Verification items for the finished model (mm, model axes). A direction names the side the tool comes from. Coordinates: 2 decimals unless noted, no trailing zeros. Answer as a JSON object with one key per item and string values. Group by question number.
Q1. Cross-section at A-A on x = -26. Give the number of separate pieces and of enclosed holes in the cut face, and give its area (3 significant figures).
Q2. Scan lines: L1, parallel to Y at x = -3, z = 2.25; L2, parallel to X at y = -32, z = 1; L3, parallel to X at y = 7.5, z = 1.75. Record each from-to range of solid material in increasing order.
Q3. Set-up check for faces 1 (the flat face through (24, 11, 1.27)), 2 (the flat face through (-18.442, 15.377, -0.662)): record each of +Z, -Z, +X, -X, +Y, -Y from which the full face is reachable in a straight line by a thin tool's end or side.
Q4. Gauge pin test, flat ends, axial feed: pin 1 Ø6 at (x, y) = (-15.5, -22) entering from +Z; pin 2 Ø1.1 at (y, z) = (22.5, 0) entering from -X; pin 3 Ø1.5 at (y, z) = (22.5, -1) entering from +X. Record the tip position at first contact, or that the pin passes through.
Q5. Release check for a two-part mould opening along Y. For faces 3 (the cylindrical face through (42.397, 13.352, 3.102)), 4 (the flat face through (0, -2, 3.81)), 5 (the flat face through (-15, -21, 1.27)) record: released by +Y, released by -Y, zero draft, split by the parting line, or undercut.
```python
from build123d import *

# Parameters (mm, degrees)
BOSS_EXTRUDE1_DEPTH        = 3.81
BOSS_EXTRUDE1_DEPTH_BACK   = 2.54
SKETCH1_R                  = 44.45
SKETCH1_R_2                = 38.1
BOSS_EXTRUDE1_2_DEPTH      = 3.81
BOSS_EXTRUDE1_2_DEPTH_BACK = 2.54
SKETCH1_R_3                = 9.525
BOSS_EXTRUDE2_DEPTH        = 1.27
BOSS_EXTRUDE2_DEPTH_BACK   = 2.54
CUT_EXTRUDE1_DEPTH         = 5.08
CUT_EXTRUDE1_DEPTH_BACK    = 5.08
SKETCH4_R                  = 1.5875
SKETCH6_R                  = 1.778


with BuildPart() as part:
    # Sketch1 → Boss-Extrude1 (new, two sides: drawn at the far end of the back side and taken through both)
    with BuildSketch(Plane.XY.offset(-BOSS_EXTRUDE1_DEPTH_BACK)):
        Circle(SKETCH1_R)
        Circle(SKETCH1_R_2, mode=Mode.SUBTRACT)
    extrude(amount=BOSS_EXTRUDE1_DEPTH + BOSS_EXTRUDE1_DEPTH_BACK)



with BuildPart() as body_2:
    # Sketch1 → Boss-Extrude1 2 (new, two sides: drawn at the far end of the back side and taken through both)
    with BuildSketch(Plane.XY.offset(-BOSS_EXTRUDE1_2_DEPTH_BACK)):
        Circle(SKETCH1_R_3)
        with BuildLine():
            Line((-1.344041666, 1.524), (1.344041666, 1.524))
            ThreePointArc((1.344041666, 1.524), (2.032, 0), (1.344041666, -1.524))
            Line((1.344041666, -1.524), (-1.344041666, -1.524))
            ThreePointArc((-1.344041666, -1.524), (-2.032, 0), (-1.344041666, 1.524))
        make_face(mode=Mode.SUBTRACT)
    extrude(amount=BOSS_EXTRUDE1_2_DEPTH + BOSS_EXTRUDE1_2_DEPTH_BACK)


with BuildPart() as part_1:
    add(part.part)

    add(body_2.part)  # Boss-Extrude2 merges body 2
    # Sketch2 → Boss-Extrude2 (add, two sides: drawn at the far end of the back side and taken through both)
    with BuildSketch(Plane.XY.offset(-BOSS_EXTRUDE2_DEPTH_BACK)):
        with BuildLine():
            Line((0, 9.525), (0, 38.1))
            ThreePointArc((0, 38.1), (3.186160517, 37.966542918), (6.35, 37.567106623))
            Line((6.35, 37.567106623), (1.778, 9.357582006))
            Line((1.778, 9.357582006), (0, 9.525))
        make_face()
        with BuildLine():
            Line((4.7625, 8.248891971), (19.05, 32.995567884))
            ThreePointArc((19.05, 32.995567884), (21.742567407, 31.286910403), (24.282814625, 29.359068682))
            Line((24.282814625, 29.359068682), (6.218584171, 7.214903735))
            Line((6.218584171, 7.214903735), (4.7625, 8.248891971))
        make_face()
        with BuildLine():
            Line((8.248891971, 4.7625), (32.995567884, 19.05))
            ThreePointArc((32.995567884, 19.05), (34.473070919, 16.223975511), (35.709068682, 13.284291997))
            Line((35.709068682, 13.284291997), (8.992903735, 3.138997835))
            Line((8.992903735, 3.138997835), (8.248891971, 4.7625))
        make_face()
        with BuildLine():
            Line((9.525, 0), (38.1, 0))
            ThreePointArc((38.1, 0), (37.966542918, -3.186160517), (37.567106623, -6.35))
            Line((37.567106623, -6.35), (9.357582006, -1.778))
            Line((9.357582006, -1.778), (9.525, 0))
        make_face()
        with BuildLine():
            Line((8.248891971, -4.7625), (32.995567884, -19.05))
            ThreePointArc((32.995567884, -19.05), (31.286910403, -21.742567407), (29.359068682, -24.282814625))
            Line((29.359068682, -24.282814625), (7.214903735, -6.218584171))
            Line((7.214903735, -6.218584171), (8.248891971, -4.7625))
        make_face()
        with BuildLine():
            Line((4.7625, -8.248891971), (19.05, -32.995567884))
            ThreePointArc((19.05, -32.995567884), (16.223975511, -34.473070919), (13.284291997, -35.709068682))
            Line((13.284291997, -35.709068682), (3.138997835, -8.992903735))
            Line((3.138997835, -8.992903735), (4.7625, -8.248891971))
        make_face()
        with BuildLine():
            Line((0, -9.525), (0, -38.1))
            ThreePointArc((0, -38.1), (-3.186160517, -37.966542918), (-6.35, -37.567106623))
            Line((-6.35, -37.567106623), (-1.778, -9.357582006))
            Line((-1.778, -9.357582006), (0, -9.525))
        make_face()
        with BuildLine():
            Line((-4.7625, -8.248891971), (-19.05, -32.995567884))
            ThreePointArc((-19.05, -32.995567884), (-21.742567407, -31.286910403), (-24.282814625, -29.359068682))
            Line((-24.282814625, -29.359068682), (-6.218584171, -7.214903735))
            Line((-6.218584171, -7.214903735), (-4.7625, -8.248891971))
        make_face()
        with BuildLine():
            Line((-8.248891971, -4.7625), (-32.995567884, -19.05))
            ThreePointArc((-32.995567884, -19.05), (-34.473070919, -16.223975511), (-35.709068682, -13.284291997))
            Line((-35.709068682, -13.284291997), (-8.992903735, -3.138997835))
            Line((-8.992903735, -3.138997835), (-8.248891971, -4.7625))
        make_face()
        with BuildLine():
            Line((-9.525, 0), (-38.1, 0))
            ThreePointArc((-38.1, 0), (-37.966542918, 3.186160517), (-37.567106623, 6.35))
            Line((-37.567106623, 6.35), (-9.357582006, 1.778))
            Line((-9.357582006, 1.778), (-9.525, 0))
        make_face()
        with BuildLine():
            Line((-8.248891971, 4.7625), (-32.995567884, 19.05))
            ThreePointArc((-32.995567884, 19.05), (-31.286910403, 21.742567407), (-29.359068682, 24.282814625))
            Line((-29.359068682, 24.282814625), (-7.214903735, 6.218584171))
            Line((-7.214903735, 6.218584171), (-8.248891971, 4.7625))
        make_face()
        with BuildLine():
            Line((-4.7625, 8.248891971), (-19.05, 32.995567884))
            ThreePointArc((-19.05, 32.995567884), (-16.223975511, 34.473070919), (-13.284291997, 35.709068682))
            Line((-13.284291997, 35.709068682), (-3.138997835, 8.992903735))
            Line((-3.138997835, 8.992903735), (-4.7625, 8.248891971))
        make_face()
    extrude(amount=BOSS_EXTRUDE2_DEPTH + BOSS_EXTRUDE2_DEPTH_BACK)

    # Sketch4 → Cut-Extrude1 (cut, two sides: drawn at the far end of the back side and taken through both)
    with BuildSketch(Plane.XY.offset(-CUT_EXTRUDE1_DEPTH_BACK)):
        with Locations((-4.445, 4.445)):
            Circle(SKETCH4_R)
        with Locations((4.445, 4.445)):
            Circle(SKETCH4_R)
        with Locations((4.445, -4.445)):
            Circle(SKETCH4_R)
        with Locations((-4.445, -4.445)):
            Circle(SKETCH4_R)
    extrude(amount=CUT_EXTRUDE1_DEPTH + CUT_EXTRUDE1_DEPTH_BACK, mode=Mode.SUBTRACT)

    # Sketch6 → Cut-Revolve1 (revolve, cut)
    with BuildSketch(Plane(origin=(0, 0, 0), x_dir=(0, 0, -1), z_dir=(1, 0, 0)), mode=Mode.PRIVATE) as cut_revolve1_sk:
        with Locations((-0.635, 44.45)):
            Circle(SKETCH6_R)
    revolve(cut_revolve1_sk.sketch.rotate(Axis((0, 0, 17.923706186), (0, 0, -1)), 90), axis=Axis((0, 0, 17.923706186), (0, 0, -1)), mode=Mode.SUBTRACT)


solid = part_1.part
```
Computed values:
{
 "1": {"separate pieces": "5", "enclosed holes": "0", "area": "154 mm²"},
 "2": {"L1": "y = -43.6 to -37.98, -9.04 to -5.1, -3.79 to 3.79, 5.1 to 9.04, 37.98 to 43.6", "L2": "x = -28.29 to -18.48, -5.45 to 0, 11.88 to 18.48, 20.68 to 28.29", "L3": "x = -42.41 to -37.35, -5.87 to 5.87, 37.35 to 42.41"},
 "3": {"face 1": "+Z", "face 2": "+Z, -Z"},
 "4": {"pin 1": "stops at z = 1.27", "pin 2": "stops at x = -36.88", "pin 3": "stops at x = 38.76"},
 "5": {"face 3": "split by the parting line", "face 4": "zero draft", "face 5": "undercut"}
}
